Autodesk Inventor part; units mm, degrees
ref_plane "YZ Plane" through (0, 0, 0) normal (1, 0, 0) x (0, 1, 0)
ref_plane "XZ Plane" through (0, 0, 0) normal (0, 1, 0) x (-1, 0, 0)
ref_plane "XY Plane" through (0, 0, 0) normal (0, 0, 1) x (1, 0, 0)
sketch "Sketch1" plane through (0, 0, 0) normal (0, 1, 0) x (-1, 0, 0)
  line L0 (0, -85.725) -> (0, 14.2875)
  line L1 (-90.17, 0) -> (52.07, 0)
  line L2 (-50.8, -52.3875) -> (31.75, -52.3875)
  line L3 (-69.85, -71.4375) -> (31.75, -71.4375)
  line L4 (-69.85, -26.9875) -> (-50.8, -26.9875)
  line L5 (-50.8, -26.9875) -> (-50.8, -52.3875)
  line L6 (-69.85, -26.9875) -> (-69.85, -71.4375)
  line L7 (-53.975, -26.9875) -> (-66.675, -26.9875) construction
  line L8 (-66.675, -26.9875) -> (-66.675, -71.4375) construction
  line L9 (-66.675, -71.4375) -> (-53.975, -71.4375) construction
  line L10 (-53.975, -71.4375) -> (-53.975, -26.9875) construction
  line L11 (-60.325, -26.9875) -> (-60.325, -71.4375) construction
  line L12 (31.75, -52.3875) -> (31.75, -71.4375)
  point P0 (0, 0)
  dimension "d3" = 26.9875
  dimension "d5" = 19.05
  dimension "d6" = 3.175
  dimension "d7" = 50.8
  dimension "d11" = 19.05
  dimension "d57" = 101.6
  dimension "d58" = 12.7
  dimension "d59" = 44.45
extrude "Extrusion1" add sketch "Sketch1" along normal mid plane 12.7
sketch "Sketch2" plane through (0, 6.35, 0) normal (0, 1, 0) x (1, 0, 0)
  line L0 (-31.75, 52.3875) -> (50.8, 52.3875)
  line L1 (50.8, 52.3875) -> (50.8, 26.9875)
  line L2 (50.8, 26.9875) -> (69.85, 26.9875)
  line L3 (69.85, 26.9875) -> (69.85, 71.4375)
  line L4 (69.85, 71.4375) -> (-31.75, 71.4375)
  line L5 (50.8, 26.9875) -> (69.85, 26.9875)
  line L6 (69.85, 71.4375) -> (-31.75, 71.4375)
  line L7 (53.975, 26.9875) -> (66.675, 26.9875)
  line L8 (66.675, 26.9875) -> (66.675, 71.4375)
  line L9 (66.675, 71.4375) -> (53.975, 71.4375)
  line L10 (53.975, 71.4375) -> (53.975, 26.9875)
  line L11 (60.325, -63.5) -> (60.325, 99.2856) construction
  line L12 (102.235, 0) -> (-124.46, 0)
  line L13 (-31.75, 71.4375) -> (-31.75, 52.3875)
  point P0 (0, 0)
  point P1 (60.325, 26.9875)
  dimension "d60" = 12.7
  dimension "d61" = 6.35
extrude "Extrusion2" cut sketch "Sketch2" against normal blind 4.7625 contours L4 L8 L2 L10
chamfer "Chamfer1" distance 1.5875 angle 45 3 edges at (69.85, 0, -26.9875) (69.85, 0, -71.4375) (50.8, 0, -26.9875)
sketch "Sketch4" plane through (0, 1.5875, 0) normal (0, 1, 0) x (1, 0, 0)
  line L0 (53.975, 71.4375) -> (66.675, 71.4375)
  line L1 (53.975, 26.9875) -> (53.975, 71.4375)
  line L2 (66.675, 26.9875) -> (53.975, 26.9875)
  line L3 (66.675, 71.4375) -> (66.675, 26.9875)
  point P0 (0, 0)
  point P1 (60.325, 42.8625)
  dimension "d44" = 15.875
  dimension "d46" = 6.35
hole "Hole2" at (60.325, 1.5875, -42.8625) direction (0, -1, 0) diameter 3.302 end through all
chamfer "Chamfer3" distance 0.7937 angle 45 4 edges at (66.675, 3.9687, -26.9875) (53.975, 3.9687, -26.9875) (53.975, 3.9687, -71.4375) (66.675, 3.9687, -71.4375)
sketch "Sketch5" plane through (0, 6.35, 0) normal (0, 1, 0) x (1, 0, 0)
  line L0 (53.1813, 71.4375) -> (53.975, 70.6437)
  line L1 (53.1813, 71.4375) -> (-31.75, 71.4375)
  line L2 (-31.75, 71.4375) -> (-31.75, 52.3875)
  line L3 (-31.75, 52.3875) -> (50.8, 52.3875)
  line L4 (50.8, 52.3875) -> (50.8, 28.575)
  line L5 (52.3875, 26.9875) -> (50.8, 28.575)
  line L6 (52.3875, 26.9875) -> (53.1813, 26.9875)
  line L7 (53.975, 27.7812) -> (53.1813, 26.9875)
  line L8 (53.975, 27.7812) -> (53.975, 70.6437)
  line L9 (-31.75, 71.4375) -> (-31.75, 52.3875) construction
  line L10 (-31.75, 61.9125) -> (53.975, 61.9125) construction
  point P0 (0, 0)
  point P1 (-19.05, 61.9125)
  point P2 (6.35, 61.9125)
  dimension "d62" = 12.7
  dimension "d63" = 25.4
hole "Hole3" at (-19.05, 6.35, -61.9125) at (6.35, 6.35, -61.9125) direction (0, -1, 0) diameter 6.7564 end through all counterbore diameter 11.1252 counterbore depth 6.35
chamfer "Chamfer4" distance 3.175 angle 45 2 edges at (-31.75, 0, -52.3875) (-31.75, 0, -71.4375)
fillet "Fillet2" radius 6.35 1 edges at (50.8, 0, -52.3875)
ref_plane "Work Plane3" through (-28.575, -6.35, -61.9125) normal (0, 0, 1) x (1, 0, 0)
ref_plane "Work Plane4" through (60.325, -6.35, -69.85) normal (1, 0, 0) x (0, 0, -1)
equation "\"d3\" = 0.5 * d2"
equation "\"d7\" = 0.5 * d4"
equation "\"d11\" = d10"
equation "\"d61\" = 0.5 * d60"
properties part number "Holder - headbars - L - RH" material "Stainless Steel"
Can you work these out from the model? Positions are in its coordinate system, mm. A direction names the side the tool comes from. Round coordinates to 2 decimals unless told otherwise and drop trailing zeros. Loops run counter-clockwise (first coordinate to the right, second up) from the corner with the lowest first, then second, coordinate; pieces in that order, holes last. Notation, with made-up numbers: (22.25, 67) - (46.25, 67) arc R31 cw to (46.25, 96) - close; hole circle Ø11 at (81, 2). An arc over 180 degrees is marked (long way). Use CSV: the item, a comma, the result in double quotes. Start each with the question number.
1) For pin 1 Ø6 at (x, y) = (26, -4) entering from +Z; pin 2 Ø8 at (x, z) = (6.35, -61.91) entering from +Y; pin 3 Ø6.5 at (x, z) = (-19.05, -61.91) entering from -Y; pin 4 Ø2.5 at (y, z) = (4.5, -49) entering from -X, each with a flat end and sliding along its axis, tell me the tip position at first contact or that it passes through.
2) If we section it at A-A on x = -19.05: Write out the boundary of the cut face in (y, z).
3) If we section it at C-C on y = -1.75: Count the separate pieces of the cut face and the enclosed holes in it, plus the area to 3 significant figures.
4) We'd pull the mould along X, two halves only. Please class faces 4 (the flat face through (53.975, 4, -50)), 5 (the cylindrical face through (-19.199, -3.219, -65.287)), 6 (the flat face through (50.8, 0, -37)), 7 (the flat face through (69.85, 0, -49)): released by +X, released by -X, zero draft, split by the parting line, or undercut.
5) Please list where these lines run through material, in increasing order: probe 1 along X at (y, z) = (3, -57.5) (3 decimals); probe 2 along Z at (x, y) = (-19.05, -4.75); probe 3 along X at (y, z) = (-1.75, -63.5). Write a range as [from, to].
6) If we section it at D-D on x = 38: Write out the boundary of the cut face in (y, z).
7) For faces 1 (the flat face through (8, 0, -52.388)), 2 (the cylindrical face through (-16.919, 3.131, -56.774)), 3 (the cylindrical face through (6.201, -3.219, -65.287)), which set-ups out of +Z, -Z, +X, -X, +Y, -Y let a thin tool reach every point of the face, with its end or its side?
Geometry results:
1,pin 1,"stops at z = -52.39"
1,pin 2,"stops at y = 0"
1,pin 3,"passes through"
1,pin 4,"stops at x = 49.2"
2,outline,"(-6.35, -71.44) - (6.35, -71.44) - (6.35, -67.48) - (0, -67.48) - (0, -65.29) - (-6.35, -65.29) - close; (-6.35, -58.53) - (0, -58.53) - (0, -56.35) - (6.35, -56.35) - (6.35, -52.39) - (-6.35, -52.39) - close"
3,separate pieces,"1"
3,enclosed holes,"3"
3,area,"2,330 mm2"
4,face 4,"undercut"
4,face 5,"undercut"
4,face 6,"released by -X"
4,face 7,"released by +X"
5,probe 1,"x = [-31.75, -22.437], [-15.663, 2.963], [9.737, 53.975], [66.675, 69.85]"
5,probe 2,"z = [-71.44, -65.29], [-58.53, -52.39]"
5,probe 3,"x = [-31.75, -22.03], [-16.07, 3.37], [9.33, 69.85]"
6,outline,"(-6.35, -71.44) - (6.35, -71.44) - (6.35, -52.39) - (-6.35, -52.39) - close"
7,face 1,"+Z, -X, +Y, -Y"
7,face 2,"+Y"
7,face 3,"+Y, -Y"
